For this review, take the finished solid that the model builds, in its own axes (mm). Give positions to 0.01 mm unless a question says otherwise; leave off trailing zeros. Write each loop counter-clockwise with the first axis right and the second up, starting at its lowest first coordinate (ties: lowest second). Pieces come first, ordered by that corner, then holes.
from build123d import *

# Parameters (mm, degrees)
ESQUISSE1_W             = 439
ESQUISSE1_H             = 210
BOSS_EXTRU_1_DEPTH      = 3
ESQUISSE5_R             = 1.477381552
ESQUISSE5_R_2           = 1.598396888
ESQUISSE5_R_3           = 1.5875
ESQUISSE5_R_4           = 2.314661152
ENL_V_MAT_EXTRU_3_DEPTH = 4
ESQUISSE10_W            = 50
ESQUISSE10_H            = 3
ENL_V_MAT_EXTRU_5_DEPTH = 4
ENL_V_MAT_EXTRU_6_DEPTH = 244.33978302
FILLET1_R               = 40
SKETCH1_R               = 1.6
CUT_EXTRUDE1_DEPTH      = 244.33978302
SKETCH2_R               = 1.6
CUT_EXTRUDE2_DEPTH      = 244.33978302
SKETCH3_R               = 1.6
CUT_EXTRUDE3_DEPTH      = 244.33978302
SKETCH4_R               = 1.6
CUT_EXTRUDE4_DEPTH      = 244.33978302
SKETCH5_R               = 1.6
CUT_EXTRUDE5_DEPTH      = 244.33978302
SKETCH7_R               = 1.6
CUT_EXTRUDE6_DEPTH      = 244.33978302
SKETCH8_R               = 1.475
CUT_EXTRUDE7_DEPTH      = 244.33978302


with BuildPart() as part:
    # Esquisse1 → Boss.-Extru.1 (new body)
    with BuildSketch(Plane.XY):
        Rectangle(ESQUISSE1_W, ESQUISSE1_H)
    extrude(amount=BOSS_EXTRU_1_DEPTH)

    # Esquisse5 → Enlèv. mat.-Extru.3 (cut)
    with BuildSketch(Plane(origin=(0, 0, 0), x_dir=(-1, 0, 0), z_dir=(0, 0, -1))):
        with Locations((-145.216701852, 18.010439522)):
            Circle(ESQUISSE5_R)
        with Locations((-160.435580246, -32.780039682)):
            Circle(ESQUISSE5_R_2)
        with Locations((-188.38, -32.79)):
            Circle(ESQUISSE5_R_3)
        with Locations((-193.46, 19.28)):
            Circle(ESQUISSE5_R_4)
    extrude(amount=-ENL_V_MAT_EXTRU_3_DEPTH, mode=Mode.SUBTRACT)

    # Esquisse10 → Enlèv. mat.-Extru.5 (cut)
    with BuildSketch(Plane.XY.offset(3)):
        with Locations((-94.5, 103.5)):
            Rectangle(ESQUISSE10_W, ESQUISSE10_H)
        with Locations((94.5, 103.5)):
            Rectangle(ESQUISSE10_W, ESQUISSE10_H)
    extrude(amount=-ENL_V_MAT_EXTRU_5_DEPTH, mode=Mode.SUBTRACT)

    # Esquisse11 → Enlèv. mat.-Extru.6 (cut, through all)
    with BuildSketch(Plane.XY.offset(3)):
        with BuildLine():
            Line((-5, -50), (-5, 50))
            ThreePointArc((-5, 50), (0, 55), (5, 50))
            Line((5, 50), (5, -50))
            ThreePointArc((5, -50), (0, -55), (-5, -50))
        make_face()
    extrude(amount=-ENL_V_MAT_EXTRU_6_DEPTH, mode=Mode.SUBTRACT)

    # Fillet1
    fillet1_edges = [part.edges().sort_by_distance(p)[0] for p in [
        (219.5, -105, 1.5),
        (-219.5, -105, 1.5),
    ]]
    fillet(fillet1_edges, radius=FILLET1_R)

    # Sketch1 → Cut-Extrude1 (cut, through all)
    with BuildSketch(Plane(origin=(0, 0, 0), x_dir=(-1, 0, 0), z_dir=(0, 0, -1))):
        with Locations((-208, -61)):
            Circle(SKETCH1_R)
    extrude(amount=-CUT_EXTRUDE1_DEPTH, mode=Mode.SUBTRACT)

    # Sketch2 → Cut-Extrude2 (cut, through all)
    with BuildSketch(Plane(origin=(0, 0, 0), x_dir=(-1, 0, 0), z_dir=(0, 0, -1))):
        with Locations((208, -61)):
            Circle(SKETCH2_R)
        with Locations((175.5, -93.5)):
            Circle(SKETCH2_R)
    extrude(amount=-CUT_EXTRUDE2_DEPTH, mode=Mode.SUBTRACT)

    # Sketch3 → Cut-Extrude3 (cut, through all)
    with BuildSketch(Plane(origin=(0, 0, 0), x_dir=(-1, 0, 0), z_dir=(0, 0, -1))):
        with Locations((-175.5, -93.5)):
            Circle(SKETCH3_R)
    extrude(amount=-CUT_EXTRUDE3_DEPTH, mode=Mode.SUBTRACT)

    # Sketch4 → Cut-Extrude4 (cut, through all)
    with BuildSketch(Plane(origin=(0, 0, 0), x_dir=(-1, 0, 0), z_dir=(0, 0, -1))):
        with Locations((-198.5, 98)):
            Circle(SKETCH4_R)
        with Locations((-212.5, 84)):
            Circle(SKETCH4_R)
        with Locations((198.5, 98)):
            Circle(SKETCH4_R)
        with Locations((212.5, 84)):
            Circle(SKETCH4_R)
    extrude(amount=-CUT_EXTRUDE4_DEPTH, mode=Mode.SUBTRACT)

    # Sketch5 → Cut-Extrude5 (cut, through all)
    with BuildSketch(Plane(origin=(0, 0, 0), x_dir=(-1, 0, 0), z_dir=(0, 0, -1))):
        with Locations((77, 93)):
            Circle(SKETCH5_R)
        with Locations((-77, 93)):
            Circle(SKETCH5_R)
    extrude(amount=-CUT_EXTRUDE5_DEPTH, mode=Mode.SUBTRACT)

    # Sketch7 → Cut-Extrude6 (cut, through all)
    with BuildSketch(Plane(origin=(0, 0, 0), x_dir=(-1, 0, 0), z_dir=(0, 0, -1))):
        with Locations((-131.4, 32.8)):
            Circle(SKETCH7_R)
        with Locations((-159.3, 32.8)):
            Circle(SKETCH7_R)
        with Locations((-116.2, 83.6)):
            Circle(SKETCH7_R)
        with Locations((-164, 84.7)):
            Circle(SKETCH7_R)
    extrude(amount=-CUT_EXTRUDE6_DEPTH, mode=Mode.SUBTRACT)

    # Sketch8 → Cut-Extrude7 (cut, through all)
    with BuildSketch(Plane(origin=(0, 0, 0), x_dir=(-1, 0, 0), z_dir=(0, 0, -1))):
        with Locations((-98.175, -2.55)):
            Circle(SKETCH8_R)
        with Locations((-98.175, 17.45)):
            Circle(SKETCH8_R)
        with Locations((-143.675, 17.45)):
            Circle(SKETCH8_R)
        with Locations((-143.675, -2.55)):
            Circle(SKETCH8_R)
    extrude(amount=-CUT_EXTRUDE7_DEPTH, mode=Mode.SUBTRACT)


solid = part.part
(1) We need section B-B (z = 1.2). Count the separate pieces of the cut face and the enclosed holes in it, and give its area (3 significant figures).
(2) Clearance check with flat-ended pins moving along their axes: pin 1 Ø1.5 at (x, z) = (-115, 0.5) entering from +Y; pin 2 Ø2.5 at (x, y) = (77, 93) entering from +Z. State where each tip first meets the part, or that it passes through.
(3) For L1, parallel to Y at x = 175.5, z = 1.1; L2, parallel to X at y = 93, z = 2.15; L3, parallel to Y at x = 131.4, z = 1.95, list the stretches that pass through material, from the lowest coordinate up.
(4) We need section A-A (y = -11.5). Write out the cut boundary in (x, z).
The answers:
1. separate pieces: 1
1. enclosed holes: 22
1. area: 89,900 mm2
2. pin 1: stops at y = 102
2. pin 2: passes through
3. L1: y = -105 to -95.1, -91.9 to 105
3. L2: x = -219.5 to -78.6, -75.4 to 75.4, 78.6 to 219.5
3. L3: y = -105 to 31.2, 34.4 to 105
4. outline: (-219.5, 0) - (-5, 0) - (-5, 3) - (-219.5, 3) - close; (5, 0) - (219.5, 0) - (219.5, 3) - (5, 3) - close
